Check sheet for the modelled part. Datum: model origin and axes. Units: mm. Give positions to 0.01 mm unless a question says otherwise; leave off trailing zeros. Loops run counter-clockwise (first coordinate to the right, second up) from the corner with the lowest first, then second, coordinate; pieces in that order, holes last. Notation, with made-up numbers: (28.5, -5.5) - (35.5, -5.5) arc R21 cw to (35.5, 21.5) - close; hole circle Ø10 at (-28, 86). An arc over 180 degrees is marked (long way). Answer in a Markdown table with one row per item. Add a question column.
(1) Go/stop test with flat-tipped pins: P1, Ø3, axis at y = -2, z = -4, coming from the +X side; P2, Ø3, axis at y = -3, z = -3, coming from the -X side; P3, Ø1.5, axis at x = 2, z = 6.5, coming from the -Y side. Record where each tip stops, or that it passes through.
(2) Draft check along Y on faces 1 (the face through (0, 0, -9.525)), 2 (the face through (-1.926, 0.607, 3.421)), 3 (the face through (-0.86, -3.874, 0.396)). Enter one of: released by +Y, released by -Y, zero draft, split by the parting line, or undercut.
(3) Sectioned sample at B-B on z = -5.75. Enter the section's corners in (x, y), then the cut area to 3 significant figures.
(4) Thickness scan on L1, parallel to Y at x = 0, z = 2.25; L2, parallel to X at y = -1.25, z = 5.5; L3, parallel to Y at x = 1.5, z = 3.75. Record the ranges inside material, lowest first.
(5) Sectioned sample at A-A on z = 6. Enter the section's corners in (x, y), then the cut area to 3 significant figures.
from build123d import *

# Parameters (mm, degrees)
SKETCH1_R                  = 3.96875
EXTRUDE1_DEPTH             = 9.525
FILLET1_R                  = 0.254
CHAMFER1_SIZE              = 0.79375
F_10_32_TAPPED_HOLE1_D     = 4.0386
F_10_32_TAPPED_HOLE1_DEPTH = 12.0396
F_10_32_TAPPED_HOLE1_TIP   = 1.213317848


with BuildPart() as part:
    # Sketch1 → Extrude1 (new body, symmetric)
    with BuildSketch(Plane.XY):
        Circle(SKETCH1_R)
    extrude(amount=EXTRUDE1_DEPTH, both=True)

    # Fillet1
    fillet1_edges = [part.edges().sort_by_distance(p)[0] for p in [
        (-3.96875, 0, 9.525),
    ]]
    fillet(fillet1_edges, radius=FILLET1_R)

    # Chamfer1
    chamfer1_edges = [part.edges().sort_by_distance(p)[0] for p in [
        (-3.96875, 0, -9.525),
    ]]
    chamfer(chamfer1_edges, length=CHAMFER1_SIZE)

    # #10-32 Tapped Hole1
    with Locations(Plane.XY.offset(9.525)):
        with Locations((0, 0)):
            Hole(F_10_32_TAPPED_HOLE1_D / 2, depth=F_10_32_TAPPED_HOLE1_DEPTH)
            with Locations((0, 0, -(F_10_32_TAPPED_HOLE1_DEPTH + F_10_32_TAPPED_HOLE1_TIP / 2))):  # 118° drill point
                Cone(0, F_10_32_TAPPED_HOLE1_D / 2, F_10_32_TAPPED_HOLE1_TIP, mode=Mode.SUBTRACT)


solid = part.part
Reply:
| question | item | result |
|---|---|---|
| 1 | P1 | x = 3.94 |
| 1 | P2 | x = -3.67 |
| 1 | P3 | y = -3.77 |
| 2 | face 1 | zero draft |
| 2 | face 2 | undercut |
| 2 | face 3 | split by the parting line |
| 3 | outline | circle Ø7.94 at (0, 0) |
| 3 | area | 49.5 mm^2 |
| 4 | L1 | -3.97 to -2.02, 2.02 to 3.97 |
| 4 | L2 | -3.77 to -1.59, 1.59 to 3.77 |
| 4 | L3 | -3.67 to -1.35, 1.35 to 3.67 |
| 5 | outline | circle Ø7.94 at (0, 0); hole circle Ø4.04 at (0, 0) |
| 5 | area | 36.7 mm^2 |
